The model under review builds one solid part; all positions refer to its coordinate system, in mm. Coordinates: 2 decimals unless noted, no trailing zeros. Loops run counter-clockwise (first coordinate to the right, second up) from the corner with the lowest first, then second, coordinate; pieces in that order, holes last. Notation, with made-up numbers: M -23,28 L -12,28 A30 ccw -12,55 Z; hole C 89,60.5 d7. An arc over 180 degrees is marked long. Use CSV: the item, a comma, the result in double quotes. Start each with the question number.
1. Add section B-B, the plane y = 58. Write out the cut boundary in (x, z), then the cut area to 3 significant figures.
2. For L1, parallel to Y at x = 0, z = 0.45; L2, parallel to X at y = 20.5, z = 0.35; L3, parallel to Y at x = 72, z = 0.35, list the stretches that pass through material, from the lowest coordinate up.
3. Add section A-A, the plane z = 0.4. Write out the cut boundary in (x, y), then the cut area to 3 significant figures.
4. Add section C-C, the plane x = -67.5. Write out the cut boundary in (y, z), then the cut area to 3 significant figures.
from build123d import *

# Parameters (mm, degrees)
BOX_W             = 30
BOX_H             = 70
BOX_DEPTH         = 0.5
BOX001_W          = 30
BOX001_H          = 70
BOX001_DEPTH      = 0.5
CYLINDER004_R     = 0.62
CYLINDER004_DEPTH = 0.5
CYLINDER003_R     = 0.62
CYLINDER003_DEPTH = 0.5
CYLINDER001_R     = 0.62
CYLINDER001_DEPTH = 0.5
CYLINDER_R        = 80
CYLINDER_DEPTH    = 0.5


with BuildPart() as cubo:
    # Box → Box (new body)
    with BuildSketch(Plane(origin=(-80, 0, 0), x_dir=(1, 0, 0), z_dir=(0, 0, 1))):
        with Locations((15, 35)):
            Rectangle(BOX_W, BOX_H)
    extrude(amount=BOX_DEPTH)


with BuildPart() as cubo001:
    # Box001 → Box001 (new body)
    with BuildSketch(Plane(origin=(50, 0, 0), x_dir=(1, 0, 0), z_dir=(0, 0, 1))):
        with Locations((15, 35)):
            Rectangle(BOX001_W, BOX001_H)
    extrude(amount=BOX001_DEPTH)


with BuildPart() as obj1:
    # Cylinder004 → Cylinder004 (new body)
    with BuildSketch(Plane(origin=(72, -7, 0), x_dir=(1, 0, 0), z_dir=(0, 0, 1))):
        Circle(CYLINDER004_R)
    extrude(amount=CYLINDER004_DEPTH)


with BuildPart() as obj2:
    # Cylinder003 → Cylinder003 (new body)
    with BuildSketch(Plane(origin=(-72, -7, 0), x_dir=(1, 0, 0), z_dir=(0, 0, 1))):
        Circle(CYLINDER003_R)
    extrude(amount=CYLINDER003_DEPTH)


with BuildPart() as obj3:
    # Cylinder001 → Cylinder001 (new body)
    with BuildSketch(Plane(origin=(0, 72, 0), x_dir=(1, 0, 0), z_dir=(0, 0, 1))):
        Circle(CYLINDER001_R)
    extrude(amount=CYLINDER001_DEPTH)


with BuildPart() as cut004:
    # Cylinder → Cylinder (new body)
    with BuildSketch(Plane.XY):
        Circle(CYLINDER_R)
    extrude(amount=CYLINDER_DEPTH)

    # Cut: cut obj3
    add(obj3.part, mode=Mode.SUBTRACT)

    # Cut001: cut obj2
    add(obj2.part, mode=Mode.SUBTRACT)

    # Cut002: cut obj1
    add(obj1.part, mode=Mode.SUBTRACT)

    # Cut003: cut Cubo001
    add(cubo001.part, mode=Mode.SUBTRACT)

    # Cut004: cut Cubo
    add(cubo.part, mode=Mode.SUBTRACT)


solid = cut004.part
Computed:
1,outline,"M -50,0 L 50,0 L 50,0.5 L -50,0.5 Z"
1,area,"50.0 mm^2"
2,L1,"y = -80 to 71.38, 72.62 to 80"
2,L2,"x = -50 to 50"
2,L3,"y = -34.87 to -7.62, -6.38 to 0"
3,outline,"M -80,0 A80 ccw 80,0 L 50,0 L 50,62.45 A80 ccw -50,62.45 L -50,0 Z; hole C -72,-7 d1.24; hole C 0,72 d1.24; hole C 72,-7 d1.24"
3,area,"17,500 mm^2"
4,outline,"M -42.94,0 L 0,0 L 0,0.5 L -42.94,0.5 Z"
4,area,"21.5 mm^2"
